```python
from build123d import *

# Parameters (mm, degrees)
F1_DEPTH = 40
F2_W     = 28
F2_H     = 20
F3_DEPTH = 40
F5_DEPTH = 40
F2_W_2   = 3
F2_H_2   = 3
F6_DEPTH = 40


with BuildPart() as f1:
    # F0 (on Top) → F1 (new body)
    with BuildSketch(Plane.XY):
        Polygon((0, 2.385549), (20, 20), (7.583665, 20), (-9.509563, 4.945609), (-9.509563, -3.451516), (5.275408, -20), (20, -20), align=None)
        with BuildLine():
            Line((-9.509563, 4.945609), (-9.509563, 20))
            Line((-9.509563, 20), (-14, 20))
            Line((-14, 20), (-14, -15))
            ThreePointArc((-14, -15), (-15, -16), (-16, -15))
            Line((-16, -15), (-16, 20))
            Line((-16, 20), (-20, 20))
            Line((-20, 20), (-20, -20))
            Line((-20, -20), (-9.509563, -20))
            Line((-9.509563, -20), (-9.509563, -3.451516))
            Line((-9.509563, -3.451516), (-9.509563, 4.945609))
        make_face()
    extrude(amount=F1_DEPTH)

    # F2 (on face) → F3 (cut)
    with BuildSketch(Plane(origin=(-20, 0, 0), x_dir=(0, -1, 0), z_dir=(-1, 0, 0))):
        with Locations((0, 10)):
            Rectangle(F2_W, F2_H)
    extrude(amount=-F3_DEPTH, mode=Mode.SUBTRACT)

    # F4 (on face) → F5 (cut)
    with BuildSketch(Plane.XZ.offset(20)):
        Polygon((9.509967, 29.723961), (0, 20.214196), (-9.509563, 29.723961), (-9.509563, 0), (9.509967, 0), align=None)
    extrude(amount=-F5_DEPTH, mode=Mode.SUBTRACT)

    # F2 (on face) → F6 (cut)
    with BuildSketch(Plane(origin=(-20, 0, 0), x_dir=(0, -1, 0), z_dir=(-1, 0, 0))):
        with Locations((-4.974076, 32.809951)):
            Rectangle(F2_W_2, F2_H_2)
        with Locations((4.974076, 32.809951)):
            Rectangle(F2_W_2, F2_H_2)
        with Locations((-8.575957, 28.904985)):
            Rectangle(F2_W_2, F2_H_2)
        with Locations((-12.238311, 24.934458)):
            Rectangle(F2_W_2, F2_H_2)
        with Locations((8.575957, 28.904985)):
            Rectangle(F2_W_2, F2_H_2)
        with Locations((12.238311, 24.934458)):
            Rectangle(F2_W_2, F2_H_2)
    extrude(amount=-F6_DEPTH, mode=Mode.SUBTRACT)


solid = f1.part
```
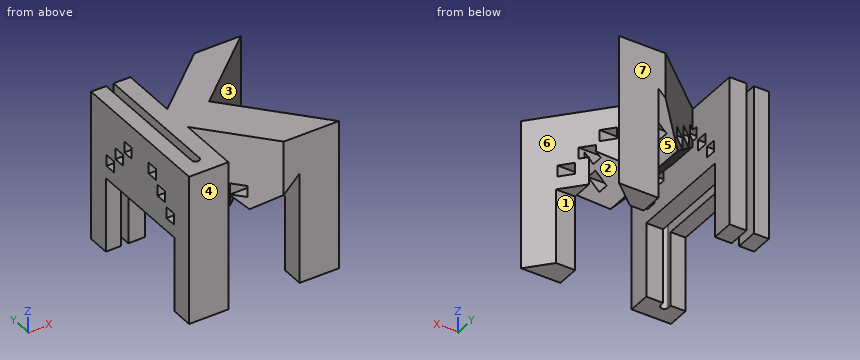
Work out the finished part from the listing and answer in its coordinate system (mm). Face numbers are marked on the shaded views. A direction names the side the tool comes from. Give positions to 0.01 mm unless a question says otherwise; leave off trailing zeros. Loops run counter-clockwise (first coordinate to the right, second up) from the corner with the lowest first, then second, coordinate; pieces in that order, holes last. Notation, with made-up numbers: (62, 24) - (68, 24) arc R11 cw to (68, 37) - close; hole circle Ø4 at (-20, 13.25). An arc over 180 degrees is marked (long way). One line per question, with ' | ' between items.
(1) The part is cut by section B-B (z = 14.5). Write down the section's boundary in (x, y).
Recorded:
outline: (-20, -20) - (-9.51, -20) - (-9.51, -14) - (-14, -14) - (-14, -15) arc R1 cw to (-16, -15) - (-16, -14) - (-20, -14) - close; (-20, 14) - (-16, 14) - (-16, 20) - (-20, 20) - close; (-14, 14) - (-9.51, 14) - (-9.51, 20) - (-14, 20) - close; (9.51, -20) - (20, -20) - (14.64, -14) - (9.51, -14) - close; (9.51, 14) - (13.19, 14) - (20, 20) - (9.51, 20) - close
(2) The mould has two halves that part along Y. Classify the marked faces 4, 5, 6 and 7: +Y half, -Y half, draft (parallel to the pull), parting line (faces both ways), or undercut.
Recorded:
face 4: -Y half | face 5: draft | face 6: undercut | face 7: +Y half
(3) The part is cut by section A-A (y = 0). Write down the section's boundary in (x, z), then the cut area to 3 significant figures.
Recorded:
outline: (-20, 20) - (-16, 20) - (-16, 40) - (-20, 40) - close; (-14, 20) - (-9.51, 20) - (-9.51, 29.72) - (0, 20.21) - (2.13, 22.35) - (2.13, 40) - (-14, 40) - close | area: 353 mm²
(4) Straight lines are drawn through the part: probe 1 along Y at (x, z) = (-13, 9.5); probe 2 along X at (y, z) = (15, 5); probe 3 along X at (y, z) = (-12, 34). For each, find the intervals that lie inside material, in ascending order.
Recorded:
probe 1: y = -20 to -14, 14 to 20 | probe 2: x = -20 to -16, -14 to -9.51, 9.51 to 14.32 | probe 3: x = -20 to -16, -14 to -9.51, -1.87 to 12.85
(5) The part is cut by section C-C (y = -5.5). Write down the section's boundary in (x, z).
Recorded:
outline: (-20, 20) - (-16, 20) - (-16, 31.31) - (-20, 31.31) - close; (-20, 34.31) - (-16, 34.31) - (-16, 40) - (-20, 40) - close; (-14, 20) - (-9.51, 20) - (-9.51, 31.31) - (-14, 31.31) - close; (-14, 34.31) - (-9.51, 34.31) - (-9.51, 40) - (-14, 40) - close; (-7.68, 27.89) - (0, 20.21) - (7.05, 27.26) - (7.05, 31.31) - (-7.68, 31.31) - close; (-7.68, 34.31) - (7.05, 34.31) - (7.05, 40) - (-7.68, 40) - close
(6) The part is cut by section D-D (z = 21). Write down the section's boundary in (x, y), then the cut area to 3 significant figures.
Recorded:
outline: (-20, -20) - (-9.51, -20) - (-9.51, 20) - (-14, 20) - (-14, -15) arc R1 cw to (-16, -15) - (-16, 20) - (-20, 20) - close; (-0.79, -13.22) - (0.79, -14.97) - (0.79, 1.51) - (0, 2.39) - (0.79, 3.08) - (0.79, 14.01) - (-0.79, 12.63) - close; (9.51, -20) - (20, -20) - (9.51, -8.26) - close; (9.51, 10.76) - (20, 20) - (9.51, 20) - close | area: 501 mm²
(7) A tool of negligible diameter and unlimited length cuts with its end or side. For the marked faces 1, 2 and 3, from which of +Z, -Z, +X, -X, +Y, -Y can it reach the whole face along a straight path? Write none if from no direction.
Recorded:
face 1: -Z, +X, -X | face 2: -Z, +Y, -Y | face 3: +Z, -Z, +X
(8) Each of these flat-tipped pins is pushed along its axis until it touches: pin 1 Ø3 at (x, y) = (-11, 8) entering from -Z; pin 2 Ø4 at (y, z) = (-4, 24) entering from +X; pin 3 Ø1 at (x, z) = (8.5, 7) entering from +Y; pin 4 Ø3.5 at (x, z) = (1.5, 28.5) entering from -Y. Where does it stop, or does it pass through?
Recorded:
pin 1: stops at z = 20 | pin 2: stops at x = 5.78 | pin 3: passes through | pin 4: stops at y = -17.73
